Print and shaded views of the part. All mm, measured from the part's lowest x, y and z. A direction names the side the tool comes from. Coordinates: 2 decimals unless noted, no trailing zeros. Order: outer loops, then holes, each group sorted by start corner. A loop starts at its lowest first (then second) coordinate and runs counter-clockwise, first axis right, second up. Notation, with made-up numbers: (35.5, -30.75) - (91.5, -30.75) arc R13 ccw to (91.5, -7.75) - close; hole circle Ø11 at (48.5, 22.25). An arc over 180 degrees is marked (long way). Write each question's results on one line, items separated by ' | '.
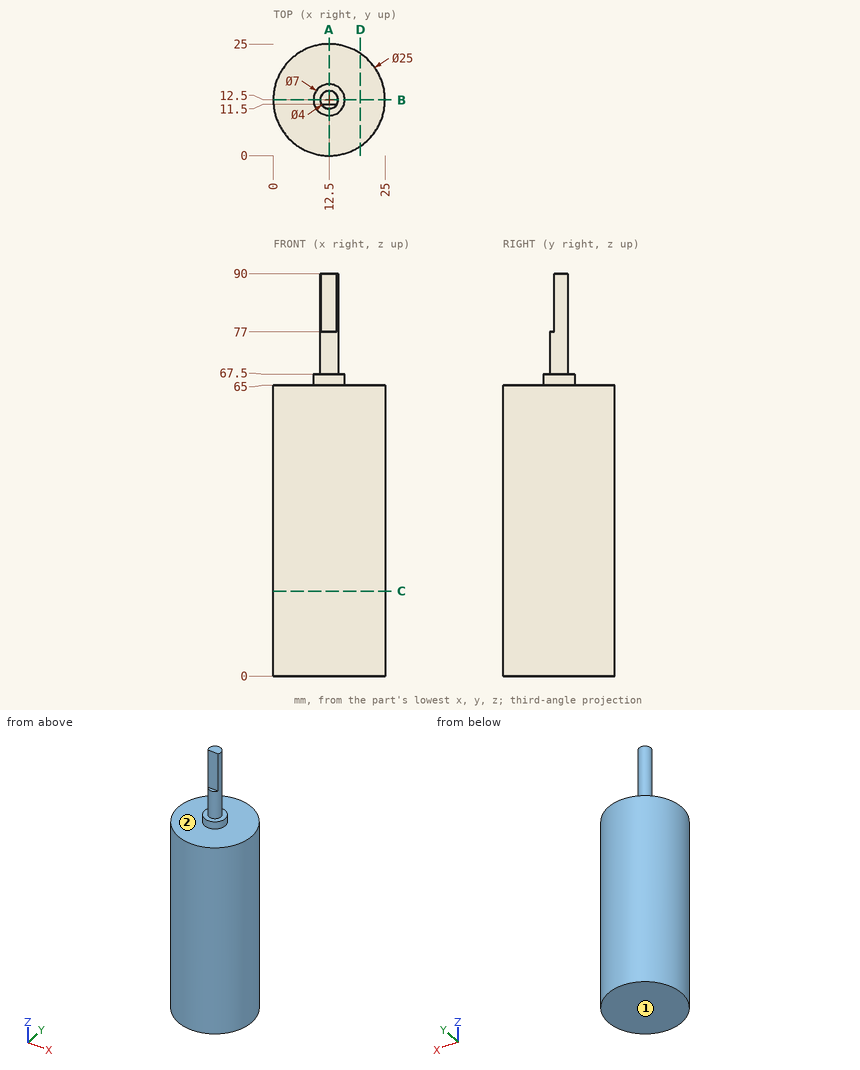
1. Drop flat-ended pins along their axis: pin 1 Ø5 at (y, z) = (10, 39) entering from +X; pin 2 Ø1 at (x, z) = (20, 12.5) entering from +Y; pin 3 Ø5 at (y, z) = (13.5, 79) entering from +X; pin 4 Ø0.8 at (x, y) = (13, 11) entering from +Z. Give the stop position or say it passes through.
Solved:
pin 1: stops at x = 25 | pin 2: stops at y = 22.86 | pin 3: stops at x = 14.5 | pin 4: stops at z = 77
2. Band-saw the part on C-C on z = 19. Give the cut face in (x, y).
Solved:
outline: circle Ø25 at (12.5, 12.5)
3. Probe line 1 (Z direction, x = 14, y = 5.25); line 2 (Y direction, x = 12, z = 29). List the from-to ranges inside material, lowest first.
Solved:
line 1: z = 0 to 65 | line 2: y = 0.01 to 24.99
4. Tool access for the marked faces 1 and 2: list every direction of +Z, -Z, +X, -X, +Y, -Y with a clear straight run to the whole face (end or side of a thin tool).
Solved:
face 1: -Z, +X, -X, +Y, -Y | face 2: +Z
5. Band-saw the part on B-B on y = 12.5. Give the cut face in (x, z), then the cut area to 3 significant figures.
Solved:
outline: (0, 0) - (25, 0) - (25, 65) - (16, 65) - (16, 67.5) - (14.5, 67.5) - (14.5, 90) - (10.5, 90) - (10.5, 67.5) - (9, 67.5) - (9, 65) - (0, 65) - close | area: 1,730 mm2
6. Band-saw the part on D-D on x = 19.5. Give the cut face in (y, z), then the cut area to 3 significant figures.
Solved:
outline: (2.14, 0) - (22.86, 0) - (22.86, 65) - (2.14, 65) - close | area: 1,350 mm2
7. Band-saw the part on A-A on x = 12.5. Give the cut face in (y, z), then the cut area to 3 significant figures.
Solved:
outline: (0, 0) - (25, 0) - (25, 65) - (16, 65) - (16, 67.5) - (14.5, 67.5) - (14.5, 90) - (11.5, 90) - (11.5, 77) - (10.5, 77) - (10.5, 67.5) - (9, 67.5) - (9, 65) - (0, 65) - close | area: 1,720 mm2
